```python
from build123d import *

# Parameters (mm, degrees)
F0_R     = 47.3075
F0_R_2   = 44.45
F1_DEPTH = 19.05
F0_R_3   = 12.7
F2_DEPTH = 50.8
F3_SIZE2 = 7.139464
F3_SIZE  = 50.79999
F4_R     = 26.9875
F4_R_2   = 12.7
F5_DEPTH = 2.921
F7_D     = 9.525
F7_DEPTH = 19.05
F7_TIP   = 2.8615986981
F8_SIZE  = 0.8128


# Not quite as in the source:
# - a fillet or chamfer is up to 0.001 mm smaller than in the source, because OpenCascade refuses the exact size


with BuildPart() as f1:
    # F0 (on Front) → F1 (new body)
    with BuildSketch(Plane.XZ):
        Circle(F0_R)
        Circle(F0_R_2, mode=Mode.SUBTRACT)
    extrude(amount=F1_DEPTH)

    # F0 (on Front) → F2 (join)
    with BuildSketch(Plane.XZ):
        Circle(F0_R_2)
        Circle(F0_R_3, mode=Mode.SUBTRACT)
    extrude(amount=F2_DEPTH)

    # F3 (size 50.8 and 7.1394744029 in the source; OpenCascade refuses exactly that, so slightly less here)
    f3_edges = [f1.edges().sort_by_distance(p)[0] for p in [
        (-12.7, 0, 0),
    ]]
    f3_side = f1.faces().sort_by_distance((-12.7, -25.4, 0))[0]
    chamfer(f3_edges, length=F3_SIZE, length2=F3_SIZE2, reference=f3_side)

    # F4 (on face) → F5 (cut)
    with BuildSketch(Plane.XZ):
        Circle(F4_R)
        Circle(F4_R_2, mode=Mode.SUBTRACT)
    extrude(amount=F5_DEPTH, mode=Mode.SUBTRACT)

    # F7
    with Locations(Plane.XZ.offset(50.8)):
        with Locations((-25.4, 25.4), (25.4, 25.4), (-25.4, -25.4), (25.4, -25.4)):
            Hole(F7_D / 2, depth=F7_DEPTH)
            with Locations((0, 0, -(F7_DEPTH + F7_TIP / 2))):  # 118° drill point
                Cone(0, F7_D / 2, F7_TIP, mode=Mode.SUBTRACT)

    # F8
    f8_edges = [f1.edges().sort_by_distance(p)[0] for p in [
        (-44.45, -50.8, 0),
        (-47.3075, -19.05, 0),
        (-47.3075, 0, 0),
    ]]
    chamfer(f8_edges, length=F8_SIZE)


solid = f1.part
```
Source: CAD feature listing. Evaluate the final solid. Frame: model axes, mm. A direction names the side the tool comes from. Coordinates: 2 decimals unless noted, no trailing zeros. Write each loop counter-clockwise with the first axis right and the second up, starting at its lowest first coordinate (ties: lowest second). Pieces come first, ordered by that corner, then holes. Notation, with made-up numbers: M 67,-25.75 L 115,-25.75 A35 cw 115,10.25 Z; hole C 82,57 d3. An arc over 180 degrees is marked long. Answer as a JSON object with one key per item and string values.
1. Contact query for flat-ended pins moving along their axis: P1, Ø1.5, axis at y = -23.5, z = 9.5, coming from the -X side; P2, Ø5.5, axis at x = 25.4, z = -25.4, coming from the -Y side; P3, Ø12, axis at y = -28.5, z = -32, coming from the +X side. Output: stop coordinate, or through.
Evaluation:
{"P1": "x = -43.58", "P2": "y = -30.54", "P3": "x = 36.05"}
2. Draft query along X for faces 1 (the flat face through (9.1, -50.8, -9.1)), 2 (the conical face through (25.782, -29.385, -26.134)), 3 (the cylindrical face through (-10.26, -9.4, -46.18)). Return one class per face: released by +X, released by -X, zero draft, split by the parting line, or undercut.
Evaluation:
{"face 1": "zero draft", "face 2": "undercut", "face 3": "split by the parting line"}
3. Cut plane C-C on y = -10.5. Output: boundary loops of the cut face in (x, z) (1 decimal), plus the area to 3 significant figures.
Evaluation:
{"outline": "C 0,0 d94.6; hole C 0,0 d36.7", "area": "5,970 mm^2"}
4. Access query for faces 4 (the cylindrical face through (-27.96, -41.142, -21.384)), 5 (the flat face through (20, 0, -20)), 6 (the cylindrical face through (-19.89, -1.44, 18.24)). Directions: +Z, -Z, +X, -X, +Y, -Y. A direction counts if a zero-diameter tool reaches every point of the face in a straight line with its end or side. Return the directions, or none.
Evaluation:
{"face 4": "-Y", "face 5": "+Z, -Z, +X, -X, +Y", "face 6": "+Y"}
5. Ray query, L1, parallel to Z at x = 0, y = -1; L2, parallel to Z at x = -25, y = -44; L3, parallel to Y at x = -16, z = 18. Return the intervals inside material, ascending.
Evaluation:
{"L1": "-47.31 to -26.99, 26.99 to 47.31", "L2": "-36.75 to -30.15, -20.65 to 20.65, 30.15 to 36.75", "L3": "-50.8 to -2.92"}
6. Cut plane B-B on y = -23. Output: boundary loops of the cut face in (x, z).
Evaluation:
{"outline": "C 0,0 d88.9; hole C 0,0 d33.21"}
